The listing builds one solid part. Answer for the finished solid, in the listing's coordinates (mm). A direction names the side the tool comes from. Round coordinates to 2 decimals unless told otherwise and drop trailing zeros. Write each loop counter-clockwise with the first axis right and the second up, starting at its lowest first coordinate (ties: lowest second). Pieces come first, ordered by that corner, then holes. Notation, with made-up numbers: (30, 38) - (74, 38) arc R29 ccw to (74, 64) - close; hole circle Ø3 at (1, 8.5). An arc over 180 degrees is marked (long way). Use a Markdown table: item, result. Add a question column.
1) Determine the mould class of faces 3 (the cylindrical face through (-0.208, 16.586, -4.493)), 4 (the flat face through (5, 52, 0)), 5 (the flat face through (-4.5, 0, -0.1)) for opening direction Y: +Y half, -Y half, draft (parallel to the pull), parting line (faces both ways), or undercut.
2) A cutting plane is placed at B-B (z = -3). Give the vertices of the cut face in (x, y), then the cut area to 3 significant figures.
3) A tool of negligible diameter and unlimited length cuts with its end or side. For faces 1 (the flat face through (-4, 52, 0)), 2 (the cylindrical face through (4.507, 57.687, 0.195)), from which of +Z, -Z, +X, -X, +Y, -Y can it reach the whole face along a straight path? Write none if from no direction.
4) A cutting plane is placed at C-C (y = 37.5). Give the vertices of the cut face in (x, z), then the cut area to 3 significant figures.
5) A cutting plane is placed at D-D (y = 48.2). Give the vertices of the cut face in (x, z), then the cut area to 3 significant figures.
6) Find the intervals of material crossed by probe 1 along Y at (x, z) = (0, -4.45); probe 2 along Z at (x, y) = (-2.75, 71), in increasing order. Write a range as from..to.
7) A cutting plane is placed at A-A (y = 15). Give the vertices of the cut face in (x, z), then the cut area to 3 significant figures.
```python
from build123d import *

# Parameters (mm, degrees)
SKETCH_1_W          = 10
SKETCH_1_H          = 10
SKETCH_1_W_2        = 8
SKETCH_1_H_2        = 8
EXTRUDE_1_DEPTH     = 104.9
SKETCH_2_R          = 1.6
SKETCH_2_R_2        = 1.5
CUT_EXTRUDE_1_DEPTH = 106.494123059
SKETCH_3_R          = 1.5
SKETCH_3_R_2        = 2
CUT_EXTRUDE_2_DEPTH = 106.494123059


with BuildPart() as part:
    # ｽｹｯﾁ1 → 押し出し-薄板1 (new body)
    with BuildSketch(Plane(origin=(0, 0, 0), x_dir=(1, 0, 0), z_dir=(0, 1, 0))):
        Rectangle(SKETCH_1_W, SKETCH_1_H)
        Rectangle(SKETCH_1_W_2, SKETCH_1_H_2, mode=Mode.SUBTRACT)
    extrude(amount=EXTRUDE_1_DEPTH)

    # ｽｹｯﾁ2 → ｶｯﾄ - 押し出し1 (cut, through all)
    with BuildSketch(Plane.XY.offset(5)):
        with Locations((0, 5)):
            Circle(SKETCH_2_R)
        with Locations((0, 15)):
            Circle(SKETCH_2_R)
        with Locations((0, 92.95)):
            Circle(SKETCH_2_R_2)
        with Locations((0, 66.7)):
            Circle(SKETCH_2_R_2)
        with Locations((0, 99.9)):
            Circle(SKETCH_2_R_2)
    extrude(amount=-CUT_EXTRUDE_1_DEPTH, mode=Mode.SUBTRACT)

    # ｽｹｯﾁ3 → ｶｯﾄ - 押し出し2 (cut, through all)
    with BuildSketch(Plane(origin=(5, 0, 0), x_dir=(0, 0, -1), z_dir=(1, 0, 0))):
        with Locations((0, 76.2)):
            Circle(SKETCH_3_R)
        with Locations((0, 5)):
            Circle(SKETCH_3_R)
        with Locations((0, 64.7)):
            Circle(SKETCH_3_R_2)
        with Locations((0, 29.7)):
            Circle(SKETCH_3_R_2)
        with Locations((0, 48.2)):
            Circle(SKETCH_3_R)
        with Locations((0, 56.2)):
            Circle(SKETCH_3_R)
    extrude(amount=-CUT_EXTRUDE_2_DEPTH, mode=Mode.SUBTRACT)


solid = part.part
```
Entries:
| question | item | result |
|---|---|---|
| 1 | face 3 | undercut |
| 1 | face 4 | draft |
| 1 | face 5 | -Y half |
| 2 | outline | (-5, 0) - (-4, 0) - (-4, 104.9) - (-5, 104.9) - close; (4, 0) - (5, 0) - (5, 104.9) - (4, 104.9) - close |
| 2 | area | 210 mm² |
| 3 | face 1 | +Y, -Y |
| 3 | face 2 | +X, -X |
| 4 | outline | (-5, -5) - (5, -5) - (5, 5) - (-5, 5) - close; hole (-4, -4) - (4, -4) - (4, 4) - (-4, 4) - close |
| 4 | area | 36.0 mm² |
| 5 | outline | (-5, -5) - (5, -5) - (5, -1.5) - (4, -1.5) - (4, -4) - (-4, -4) - (-4, -1.5) - (-5, -1.5) - close; (-5, 1.5) - (-4, 1.5) - (-4, 4) - (4, 4) - (4, 1.5) - (5, 1.5) - (5, 5) - (-5, 5) - close |
| 5 | area | 30.0 mm² |
| 6 | probe 1 | y = 0..3.4, 6.6..13.4, 16.6..65.2, 68.2..91.45, 94.45..98.4, 101.4..104.9 |
| 6 | probe 2 | z = -5..-4, 4..5 |
| 7 | outline | (-5, -5) - (-1.6, -5) - (-1.6, -4) - (-4, -4) - (-4, 4) - (-1.6, 4) - (-1.6, 5) - (-5, 5) - close; (1.6, -5) - (5, -5) - (5, 5) - (1.6, 5) - (1.6, 4) - (4, 4) - (4, -4) - (1.6, -4) - close |
| 7 | area | 29.6 mm² |
